from build123d import *

# Parameters (mm, degrees)
SKETCH_1_W          = 100
SKETCH_1_H          = 99
EXTRUDE_1_DEPTH     = 3
SKETCH_2_R          = 6
SKETCH_2_R_2        = 1.6
CUT_EXTRUDE_1_DEPTH = 3
SKETCH_4_W          = 131.961579061
SKETCH_4_H          = 16.810392237
CUT_EXTRUDE_2_DEPTH = 1
M3X0_5_4_D          = 2.5
M3X0_5_4_DEPTH      = 8.5
M3X0_5_4_TIP        = 0.751075774
M3X0_5_5_D          = 2.5
M3X0_5_5_DEPTH      = 8.5
M3X0_5_5_TIP        = 0.751075774
SKETCH_11_R         = 1.6
CUT_EXTRUDE_3_DEPTH = 10
SKETCH_12_R         = 1.6
CUT_EXTRUDE_4_DEPTH = 10


with BuildPart() as part:
    # ｽｹｯﾁ1 → ﾎﾞｽ - 押し出し1 (new body)
    with BuildSketch(Plane.XY):
        Rectangle(SKETCH_1_W, SKETCH_1_H)
    extrude(amount=EXTRUDE_1_DEPTH)

    # ｽｹｯﾁ2 → ｶｯﾄ - 押し出し1 (cut)
    with BuildSketch(Plane.XY.offset(3)):
        with Locations((-18.25, -20)):
            Circle(SKETCH_2_R)
        with Locations((18.25, -20)):
            Circle(SKETCH_2_R)
        with Locations((0, 40)):
            Circle(SKETCH_2_R_2)
    extrude(amount=-CUT_EXTRUDE_1_DEPTH, mode=Mode.SUBTRACT)

    # ｽｹｯﾁ4 → ｶｯﾄ - 押し出し2 (cut)
    with BuildSketch(Plane(origin=(0, -49.5, 0), x_dir=(-1, 0, 0), z_dir=(0, -1, 0))):
        with Locations((0.945584564, -1.132272669)):
            Rectangle(SKETCH_4_W, SKETCH_4_H)
    extrude(amount=-CUT_EXTRUDE_2_DEPTH, mode=Mode.SUBTRACT)

    # M3x0.5 ねじ穴4
    with Locations(Plane(origin=(25, -43.5, 3), x_dir=(1, 0, 0), z_dir=(0, 0, 1))):
        with Locations((0, 0), (-50, 0)):
            Hole(M3X0_5_4_D / 2, depth=M3X0_5_4_DEPTH)
            with Locations((0, 0, -(M3X0_5_4_DEPTH + M3X0_5_4_TIP / 2))):  # 118° drill point
                Cone(0, M3X0_5_4_D / 2, M3X0_5_4_TIP, mode=Mode.SUBTRACT)

    # M3x0.5 ねじ穴5
    with Locations(Plane(origin=(44.122623141, 9.934763699, 0), x_dir=(-1, 0, 0), z_dir=(0, 0, -1))):
        with Locations((0, 0), (19.282623141, 15.065236301)):
            Hole(M3X0_5_5_D / 2, depth=M3X0_5_5_DEPTH)
            with Locations((0, 0, -(M3X0_5_5_DEPTH + M3X0_5_5_TIP / 2))):  # 118° drill point
                Cone(0, M3X0_5_5_D / 2, M3X0_5_5_TIP, mode=Mode.SUBTRACT)

    # ｽｹｯﾁ11 → ｶｯﾄ - 押し出し3 (cut)
    with BuildSketch(Plane(origin=(0, 0, 0), x_dir=(-1, 0, 0), z_dir=(0, 0, -1))):
        with Locations((18.25, 10)):
            Circle(SKETCH_11_R)
        with Locations((-18.25, 10)):
            Circle(SKETCH_11_R)
    extrude(amount=-CUT_EXTRUDE_3_DEPTH, mode=Mode.SUBTRACT)

    # ｽｹｯﾁ12 → ｶｯﾄ - 押し出し4 (cut)
    with BuildSketch(Plane(origin=(0, 0, 0), x_dir=(-1, 0, 0), z_dir=(0, 0, -1))):
        with Locations((-39.3, 40)):
            Circle(SKETCH_12_R)
        with Locations((39.3, 40)):
            Circle(SKETCH_12_R)
    extrude(amount=-CUT_EXTRUDE_4_DEPTH, mode=Mode.SUBTRACT)


solid = part.part
For this review, take the finished solid that the model builds, in its own axes (mm). Round coordinates to 2 decimals unless told otherwise and drop trailing zeros. Order: outer loops, then holes, each group sorted by start corner. A loop starts at its lowest first (then second) coordinate and runs counter-clockwise, first axis right, second up. Notation, with made-up numbers: (56, 62.25) -> (98, 62.25) arc R19 cw to (98, 81.25) -> close; hole circle Ø3 at (-31, 64.25). An arc over 180 degrees is marked (long way). Write item = value, one per line. Start each with the question number.
1) Take a section at B-B on y = 40. State the section outline as (x, z) points, plus the area to 3 significant figures.
2) To check wall thickness, follow line 1 (Y direction, x = 25, z = 2.05); line 2 (Y direction, x = 0, z = 1.65); line 3 (Y direction, x = -25, z = 2.1). State the ranges of each line that lie inside material, in increasing order. Write a range as from..to.
3) Take a section at C-C on y = -20. State the section outline as (x, z) points, plus the area to 3 significant figures.
4) Take a section at A-A on x = 39.3. State the section outline as (y, z) points, plus the area to 3 significant figures.
5) Take a section at D-D on x = 22. State the section outline as (y, z) points, plus the area to 3 significant figures.
6) The part is to be moulded in two halves that separate along X. For faces 1 (the face through (-1, 1, 3)), 2 (the face through (-24.84, -42.26, 1.48)), 3 (the face through (50, 0, 1)), 4 (the face through (-17, 9, 1)), say which applies: +X half, -X half, draft (parallel to the pull), parting line (faces both ways), or undercut.
Verdict:
q1.outline = (-50, 0) -> (-40.9, 0) -> (-40.9, 3) -> (-50, 3) -> close; (-37.7, 0) -> (-1.6, 0) -> (-1.6, 3) -> (-37.7, 3) -> close; (1.6, 0) -> (37.7, 0) -> (37.7, 3) -> (1.6, 3) -> close; (40.9, 0) -> (50, 0) -> (50, 3) -> (40.9, 3) -> close
q1.area = 271 mm2
q2.line_1 = -48.5..-44.75, -42.25..23.76, 26.24..49.5
q2.line_2 = -48.5..38.4, 41.6..49.5
q2.line_3 = -48.5..-44.75, -42.25..49.5
q3.outline = (-50, 0) -> (-24.25, 0) -> (-24.25, 3) -> (-50, 3) -> close; (-12.25, 0) -> (12.25, 0) -> (12.25, 3) -> (-12.25, 3) -> close; (24.25, 0) -> (50, 0) -> (50, 3) -> (24.25, 3) -> close
q3.area = 228 mm2
q4.outline = (-48.5, 0) -> (38.4, 0) -> (38.4, 3) -> (-48.5, 3) -> close; (41.6, 0) -> (49.5, 0) -> (49.5, 3) -> (41.6, 3) -> close
q4.area = 284 mm2
q5.outline = (-48.5, 0) -> (-24.68, 0) -> (-24.68, 3) -> (-48.5, 3) -> close; (-15.32, 0) -> (49.5, 0) -> (49.5, 3) -> (-15.32, 3) -> close
q5.area = 266 mm2
q6.face_1 = draft
q6.face_2 = undercut
q6.face_3 = +X half
q6.face_4 = undercut
